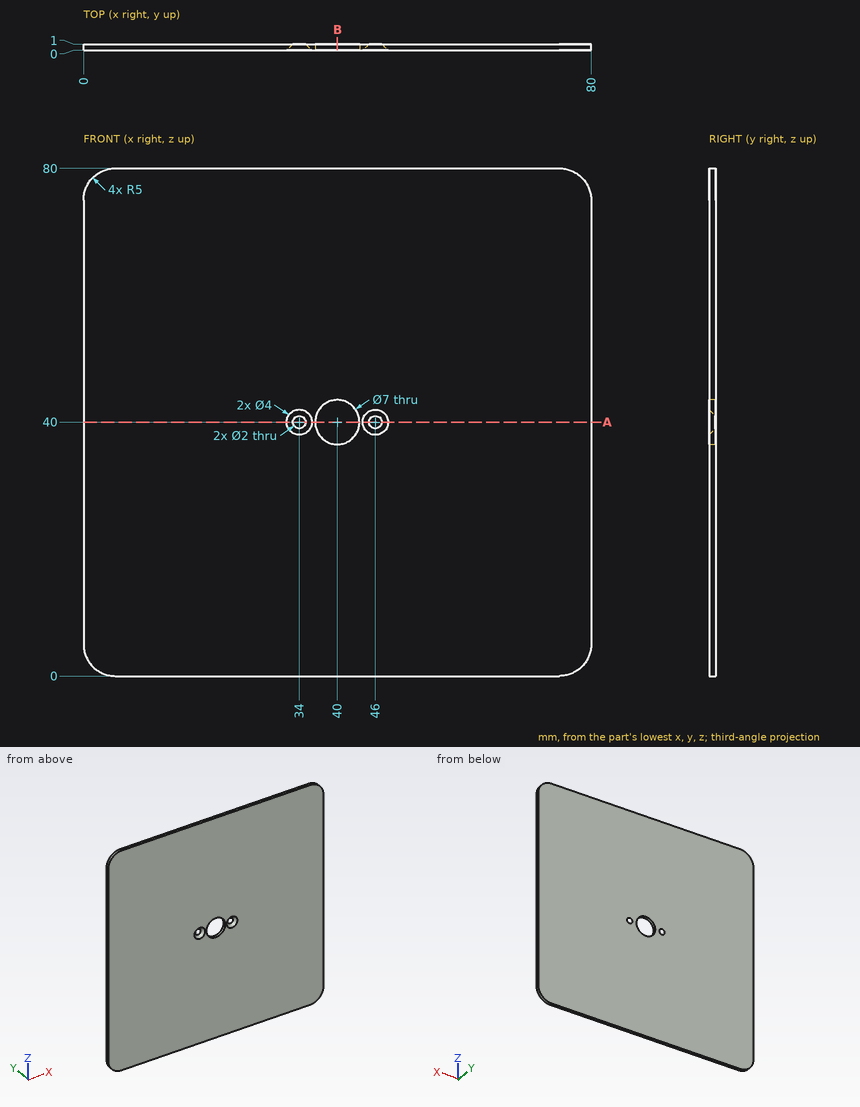
For this review, use the dimensioned drawing (mm, ordinates from the lowest corner) and the shaded views. Round coordinates to 2 decimals unless told otherwise and drop trailing zeros. Write each loop counter-clockwise with the first axis right and the second up, starting at its lowest first coordinate (ties: lowest second). Pieces come first, ordered by that corner, then holes. Notation, with made-up numbers: (-9.75, 43) -> (44.25, 43) arc R22 cw to (44.25, 56) -> close; hole circle Ø11 at (61, 86.25). An arc over 180 degrees is marked (long way). Use CSV: the item, a comma, the result in double quotes.
Q1. Consider section B-B (x = 40). Give the boundary of the cut face in (y, z).
Checks:
outline,"(0, 0) -> (1, 0) -> (1, 36.5) -> (0, 36.5) -> close; (0, 43.5) -> (1, 43.5) -> (1, 80) -> (0, 80) -> close"
Q2. To check wall thickness, follow probe 1 along X at (y, z) = (0.5, 40); probe 2 along Z at (x, y) = (38, 0.2); probe 3 along X at (y, z) = (0.2, 3). State the ranges of each line that lie inside material, in increasing order. Write a range as [from, to].
Checks:
probe 1,"[0, 32.5], [35.5, 36.5], [43.5, 44.5], [47.5, 80]"
probe 2,"[0, 37.13], [42.87, 80]"
probe 3,"[0.42, 79.58]"
Q3. Consider section A-A (z = 40). State how many separate pieces and enclosed holes the cut face has.
Checks:
separate pieces,"4"
enclosed holes,"0"
